Autodesk Inventor part; units mm, degrees
ref_plane "YZ Plane" through (0, 0, 0) normal (1, 0, 0) x (0, 1, 0)
ref_plane "XZ Plane" through (0, 0, 0) normal (0, 1, 0) x (-1, 0, 0)
ref_plane "XY Plane" through (0, 0, 0) normal (0, 0, 1) x (1, 0, 0)
sketch "Profile" plane through (0, 0, 0) normal (0, 0, 1) x (1, 0, 0)
  circle A0 centre (1024.5892, 81.5101) radius 1.27
  circle A1 centre (869.1584, 103.2274) radius 1.27
  circle A2 centre (869.1584, 121.6106) radius 1.27
  circle A3 centre (967.608, 135.3677) radius 1.27
  circle A4 centre (1024.5892, 112.7794) radius 1.27
  line L0 (963.5286, 137.2438) -> (964.6303, 134.266)
  arc A5 (964.6303, 134.266) -> (970.5595, 134.1976) centre (967.608, 135.3677) ccw
  line L1 (970.5595, 134.1976) -> (971.7296, 137.1492)
  line L2 (1022.8077, 116.901) -> (971.7296, 137.1492)
  line L3 (1022.8077, 116.901) -> (1021.6376, 113.9494)
  arc A6 (1021.6376, 113.9494) -> (1024.5892, 109.6044) centre (1024.5892, 112.7794) ccw
  line L4 (1024.5892, 109.6044) -> (1027.7642, 109.6044)
  line L5 (1027.7642, 84.6851) -> (1027.7642, 109.6044)
  line L6 (1027.7642, 84.6851) -> (1024.5892, 84.6851)
  arc A7 (1024.5892, 84.6851) -> (1021.6376, 82.6802) centre (1024.5892, 81.5101) ccw
  line L7 (1021.6376, 82.6802) -> (1020.4676, 79.7286)
  line L8 (970.7004, 99.4571) -> (1020.4676, 79.7286)
  arc A8 (970.7004, 99.4571) -> (967.5834, 100.0524) centre (967.5834, 91.5942) ccw
  line L9 (872.3334, 100.0524) -> (967.5834, 100.0524)
  line L10 (872.3334, 100.0524) -> (872.3334, 103.2274)
  arc A9 (872.3334, 103.2274) -> (869.1584, 106.4024) centre (869.1584, 103.2274) ccw
  line L11 (869.1584, 106.4024) -> (865.9834, 106.4024)
  line L12 (865.9834, 118.4356) -> (865.9834, 106.4024)
  line L13 (865.9834, 118.4356) -> (869.1584, 118.4356)
  arc A10 (869.1584, 118.4356) -> (872.3334, 121.6106) centre (869.1584, 121.6106) ccw
  line L14 (872.3334, 121.6106) -> (872.3334, 124.7856)
  line L15 (929.2861, 124.7856) -> (872.3334, 124.7856)
  arc A11 (929.2861, 124.7856) -> (930.3878, 124.9829) centre (929.2861, 127.9606) ccw
  line L16 (963.5286, 137.2438) -> (930.3878, 124.9829)
  line L17 (869.1584, 127.9606) -> (929.2861, 127.9606)
  arc A12 (869.1584, 127.9606) -> (862.8084, 121.6106) centre (869.1584, 121.6106) ccw
  line L18 (862.8084, 103.2274) -> (862.8084, 121.6106)
  arc A13 (862.8084, 103.2274) -> (869.1584, 96.8774) centre (869.1584, 103.2274) ccw
  line L19 (967.5834, 96.8774) -> (869.1584, 96.8774)
  arc A14 (969.5304, 96.5056) -> (967.5834, 96.8774) centre (967.5834, 91.5942) ccw
  line L20 (1022.2491, 75.607) -> (969.5304, 96.5056)
  arc A15 (1022.2491, 75.607) -> (1030.9392, 81.5101) centre (1024.5892, 81.5101) ccw
  line L21 (1030.9392, 112.7794) -> (1030.9392, 81.5101)
  arc A16 (1030.9392, 112.7794) -> (1026.9292, 118.6825) centre (1024.5892, 112.7794) ccw
  line L22 (969.9481, 141.2708) -> (1026.9292, 118.6825)
  arc A17 (969.9481, 141.2708) -> (965.4047, 141.3232) centre (967.608, 135.3677) ccw
  line L23 (929.2861, 127.9606) -> (965.4047, 141.3232)
  point P0 (0, 0)
extrude "ProfileFeature" add sketch "Profile" along normal blind 2.54 contours L0 A5 L1 L2 L3 A6 L4 L5 L6 A7 L7 L8 A8 L9 L10 A9 L11 L12 L13 A10 L14 L15 A11 L16 | L17 L23 A17 L22 A16 L21 A15 L20 A14 L19 A13 L18 A12
properties part number "switchback-secondary-cover"
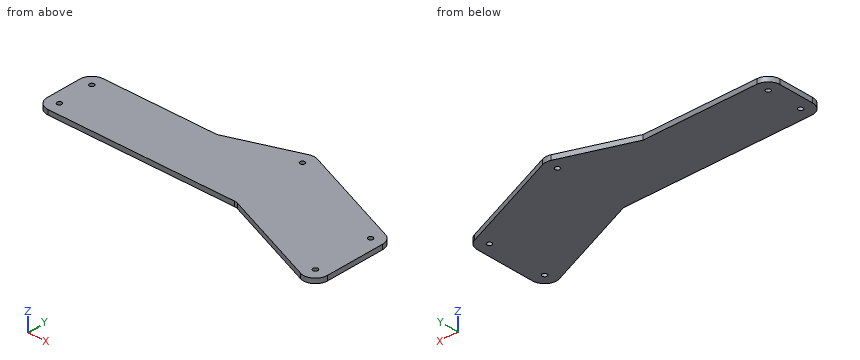
Geometry check sheet. Reference: the model listing, model coordinates, mm. Give positions to 0.01 mm unless a question says otherwise; leave off trailing zeros. Order: outer loops, then holes, each group sorted by start corner. A loop starts at its lowest first (then second) coordinate and runs counter-clockwise, first axis right, second up. Notation, with made-up numbers: M 4,38 L 30,38 A33 ccw 30,73 Z; hole C 27.5,33 d11. An arc over 180 degrees is marked long. Use a Markdown table: item, result.
Item 1: Section check B-B (x = 923). Record the cut outline in (y, z), and give its area (3 significant figures).
Answers follow:
| item | result |
|---|---|
| outline | M 96.88,0 L 127.96,0 L 127.96,2.54 L 96.88,2.54 Z |
| area | 79.0 mm2 |
Item 2: Section check A-A (z = 1.25). Record the cut outline in (x, y).
Answers follow:
| item | result |
|---|---|
| outline | M 862.81,103.23 A6.35 ccw 869.16,96.88 L 967.58,96.88 A5.28 cw 969.53,96.51 L 1022.25,75.61 A6.35 ccw 1030.94,81.51 L 1030.94,112.78 A6.35 ccw 1026.93,118.68 L 969.95,141.27 A6.35 ccw 965.4,141.32 L 929.29,127.96 L 869.16,127.96 A6.35 ccw 862.81,121.61 Z; hole C 869.16,103.23 d2.54; hole C 869.16,121.61 d2.54; hole C 967.61,135.37 d2.54; hole C 1024.59,81.51 d2.54; hole C 1024.59,112.78 d2.54 |
Item 3: Material ranges on line 1 along X through (y, z) = (112.5, 0.75); line 2 along Y through (x, z) = (880, 2.45); line 3 along Y through (x, z) = (992, 1), recorded low to high.
Answers follow:
| item | result |
|---|---|
| line 1 | x = 862.81 to 1023.35, 1025.83 to 1030.94 |
| line 2 | y = 96.88 to 127.96 |
| line 3 | y = 87.6 to 132.53 |
Item 4: Section check C-C (y = 89.5). Record the cut outline in (x, z).
Answers follow:
| item | result |
|---|---|
| outline | M 987.2,0 L 1030.94,0 L 1030.94,2.54 L 987.2,2.54 Z |
Item 5: Depth check by flat-ended pin: P1, Ø1.5, axis at x = 967.61, y = 135.37, coming from the -Z side; P2, Ø1.3, axis at x = 900.5, z = 1.5, coming from the -Y side; P3, Ø0.8, axis at x = 905.5, z = 1.5, coming from the +Y side. Enter the tip coordinate at first touch or a pass-through.
Answers follow:
| item | result |
|---|---|
| P1 | passes through |
| P2 | stops at y = 96.88 |
| P3 | stops at y = 127.96 |
